CAD build for the part. Positions are in the model's coordinates, mm. Coordinates: 2 decimals unless noted, no trailing zeros. Loops run counter-clockwise (first coordinate to the right, second up) from the corner with the lowest first, then second, coordinate; pieces in that order, holes last. Notation, with made-up numbers: (-3.75, 76.25) -> (43.25, 76.25) arc R27 ccw to (43.25, 100.25) -> close; hole circle Ø4 at (50.25, -22). An arc over 180 degrees is marked (long way). Write each question's results on one line, items separated by ' | '.
from build123d import *

# Parameters (mm, degrees)
F0_R     = 2.286
F1_DEPTH = 2.54


with BuildPart() as f1:
    # F0 (on Top) → F1 (new body)
    with BuildSketch(Plane.XY):
        with BuildLine():
            Line((0, 4.826), (-215.9, 4.826))
            ThreePointArc((-215.9, 4.826), (-220.726, 0), (-215.9, -4.826))
            Line((-215.9, -4.826), (-114.675652, -4.826))
            ThreePointArc((-114.675652, -4.826), (-112.944357, -5.147236), (-111.443546, -6.06818))
            Line((-111.443546, -6.06818), (-3.232106, -103.65982))
            ThreePointArc((-3.232106, -103.65982), (1.961139, -104.485559), (4.826, -100.076))
            Line((4.826, -100.076), (4.826, 0))
            ThreePointArc((4.826, 0), (3.412497, 3.412497), (0, 4.826))
        make_face()
        with Locations((0, -100.076)):
            Circle(F0_R, mode=Mode.SUBTRACT)
        with BuildLine():
            ThreePointArc((-215.9, -2.286), (-218.186, 0), (-215.9, 2.286))
            Line((-215.9, 2.286), (-139.7, 2.286))
            ThreePointArc((-139.7, 2.286), (-137.414, 0), (-139.7, -2.286))
            Line((-139.7, -2.286), (-215.9, -2.286))
        make_face(mode=Mode.SUBTRACT)
        with BuildLine():
            Line((-12.884106, -81.957602), (-89.084106, -13.23582))
            ThreePointArc((-89.084106, -13.23582), (-90.356764, -7.920706), (-85.852, -4.826))
            Line((-85.852, -4.826), (-9.652, -4.826))
            ThreePointArc((-9.652, -4.826), (-6.239503, -6.239503), (-4.826, -9.652))
            Line((-4.826, -9.652), (-4.826, -78.373782))
            ThreePointArc((-4.826, -78.373782), (-7.690861, -82.783341), (-12.884106, -81.957602))
        make_face(mode=Mode.SUBTRACT)
        Circle(F0_R, mode=Mode.SUBTRACT)
    extrude(amount=F1_DEPTH)


solid = f1.part
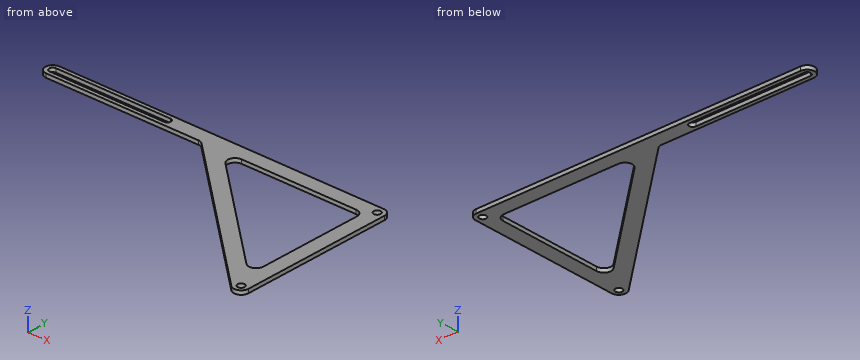
1) Slice it at A-A (x = -183.5). Write the cut outline in (y, z), then the cut area to 3 significant figures.
Outcome:
outline: (-4.83, 0) -> (-2.29, 0) -> (-2.29, 2.54) -> (-4.83, 2.54) -> close; (2.29, 0) -> (4.83, 0) -> (4.83, 2.54) -> (2.29, 2.54) -> close | area: 12.9 mm^2
2) Pin check, flat tips, straight feed: pin 1 (0.8 mm diameter, centred on x = -195, z = 2, fed in from -Y); pin 2 (12 mm diameter, centred on x = -136, y = -14.5, fed in from +Z). Stop position of each tip, or through.
Outcome:
pin 1: stops at y = -4.83 | pin 2: passes through
3) Drill centre lines: L1, parallel to Y at x = 0, z = 2.05; L2, parallel to Y at x = -211, z = 0.9; L3, parallel to X at y = 0.5, z = 2.4. Where is each one in solid material? Low to high. Write a range as from..to.
Outcome:
L1: y = -104.9..-102.36, -97.79..-2.29, 2.29..4.83 | L2: y = -4.83..-2.29, 2.29..4.83 | L3: x = -220.7..-218.13, -137.47..-2.23, 2.23..4.8
4) Slice it at B-B (y = -17.5). Write the cut outline in (x, z), then the cut area to 3 significant figures.
Outcome:
outline: (-98.77, 0) -> (-84.36, 0) -> (-84.36, 2.54) -> (-98.77, 2.54) -> close; (-4.83, 0) -> (4.83, 0) -> (4.83, 2.54) -> (-4.83, 2.54) -> close | area: 61.1 mm^2
5) Slice it at D-D (x = -103). Write the cut outline in (y, z).
Outcome:
outline: (-13.68, 0) -> (4.83, 0) -> (4.83, 2.54) -> (-13.68, 2.54) -> close
6) Slice it at C-C (z = 1.8). Write the cut outline in (x, y).
Outcome:
outline: (-215.9, -4.83) -> (-114.68, -4.83) arc R4.83 cw to (-111.44, -6.07) -> (-3.23, -103.66) arc R4.83 ccw to (4.83, -100.08) -> (4.83, 0) arc R4.83 ccw to (0, 4.83) -> (-215.9, 4.83) arc R4.83 ccw to start; hole (-215.9, -2.29) -> (-139.7, -2.29) arc R2.29 ccw to (-139.7, 2.29) -> (-215.9, 2.29) arc R2.29 ccw to start; hole (-89.08, -13.24) -> (-12.88, -81.96) arc R4.83 ccw to (-4.83, -78.37) -> (-4.83, -9.65) arc R4.83 ccw to (-9.65, -4.83) -> (-85.85, -4.83) arc R4.83 ccw to start; hole circle Ø4.57 at (0, -100.08); hole circle Ø4.57 at (0, 0)
